Geometry: final body of the model. Coordinates: model frame, mm. A direction names the side the tool comes from. Coordinates: 2 decimals unless noted, no trailing zeros. Write each loop counter-clockwise with the first axis right and the second up, starting at its lowest first coordinate (ties: lowest second). Pieces come first, ordered by that corner, then holes. Notation, with made-up numbers: (14.5, 74.25) - (35.5, 74.25) arc R21 ccw to (35.5, 108.25) - close; hole circle Ø9 at (34, 20). An arc over 180 degrees is marked (long way). Put each result on its own line as item: value.
```python
from build123d import *

# Parameters (mm, degrees)
F3_DEPTH = 2


with BuildPart() as f1:
    # F0 (on Right) → F1 (revolve)
    with BuildSketch(Plane.YZ):
        Polygon((-38, 0), (0, 0), (0, 11.925), (-23.5, 11.925), (-23.5, 9.45), (-27, 9.45), (-27, 3), (-28.5, 3), (-28.5, 0.975), (-38, 0.975), align=None)
    revolve(axis=Axis((0, -23.908602, 0), (0, -1, 0)))

    # F2 (on face) → F3 (cut)
    with BuildSketch(Plane(origin=(0, 0, 0), x_dir=(-1, 0, 0), z_dir=(0, 1, 0))):
        with BuildLine():
            Line((1.5, 11.925), (-1.5, 11.925))
            Line((-1.5, 11.925), (-1.5, 9.625))
            ThreePointArc((-1.5, 9.625), (-1.06066, 8.56434), (0, 8.125))
            ThreePointArc((0, 8.125), (1.06066, 8.56434), (1.5, 9.625))
            Line((1.5, 9.625), (1.5, 11.925))
        make_face()
        with BuildLine():
            Line((1.5, -11.925), (1.5, -9.625))
            ThreePointArc((1.5, -9.625), (0, -8.125), (-1.5, -9.625))
            Line((-1.5, -9.625), (-1.5, -11.925))
            Line((-1.5, -11.925), (1.5, -11.925))
        make_face()
    extrude(amount=-F3_DEPTH, mode=Mode.SUBTRACT)


solid = f1.part
```
1. Mould query, pull axis X, two halves, no side actions, for faces 5 (the flat face through (-9, -23.5, -4)), 6 (the cylindrical face through (-0.66, -33.32, -0.72)), 7 (the flat face through (1.5, -1, -11)). Classes: +X half, -X half, draft (parallel to the pull), parting line (faces both ways), or undercut.
Answer below:
face 5: draft
face 6: parting line
face 7: undercut
2. Pin query (flat end, axial travel): pin 1 Ø1.6 at (y, z) = (-1, 11) entering from -X; pin 2 Ø1 at (y, z) = (-0.5, -11) entering from +X; pin 3 Ø3.5 at (x, z) = (0.5, -10.5) entering from +Y; pin 4 Ø1 at (y, z) = (-20.5, 7) entering from -X. Return the tip coordinate at first contact, or that it passes through.
Answer below:
pin 1: stops at x = -6.18
pin 2: stops at x = 5.65
pin 3: stops at y = 0
pin 4: stops at x = -10
3. Set-up query: faces 1 (the flat face through (0, 0, 0)), 2 (the flat face through (1.5, -1, 11)), 3 (the flat face through (-1.5, -1, -11)), 4 (the cylindrical face through (0, -28, -3)). Return all of +Z, -Z, +X, -X, +Y, -Y with unobstructed straight access to the full face (end or side cutting, diameter ignored); none if empty.
Answer below:
face 1: +Z, -Z, +X, -X, +Y
face 2: +Z, +Y
face 3: -Z, +Y
face 4: -Y
4. Ray query, probe 1 along Y at (x, z) = (-1.75, -1.5); probe 2 along Y at (x, z) = (4.25, -7.25); probe 3 along Z at (x, y) = (0, -33.5) (3 decimals). Return the intervals inside material, ascending. Write a range as from..to.
Answer below:
probe 1: y = -28.5..0
probe 2: y = -27..0
probe 3: z = -0.975..0.975
5. Section query D-D (x = 5). Return loops of the section in (y, z), then the cut area to 3 significant figures.
Answer below:
outline: (-27, -8.02) - (-23.5, -8.02) - (-23.5, -10.83) - (0, -10.83) - (0, 10.83) - (-23.5, 10.83) - (-23.5, 8.02) - (-27, 8.02) - close
area: 565 mm²
6. Section query A-A (z = 0). Return loops of the section in (x, y) (3 decimals), then the cut area to 3 significant figures.
Answer below:
outline: (-11.925, -23.5) - (-9.45, -23.5) - (-9.45, -27) - (-3, -27) - (-3, -28.5) - (-0.975, -28.5) - (-0.975, -38) - (0.975, -38) - (0.975, -28.5) - (3, -28.5) - (3, -27) - (9.45, -27) - (9.45, -23.5) - (11.925, -23.5) - (11.925, 0) - (-11.925, 0) - close
area: 654 mm²
7. Section query B-B (x = -8.25). Return loops of the section in (y, z).
Answer below:
outline: (-27, -4.61) - (-23.5, -4.61) - (-23.5, -8.61) - (0, -8.61) - (0, 8.61) - (-23.5, 8.61) - (-23.5, 4.61) - (-27, 4.61) - close
8. Section query C-C (y = -33.5). Return loops of the section in (x, z) (3 decimals).
Answer below:
outline: circle Ø1.95 at (0, 0)
